Verification items for the finished model (mm, model axes). A direction names the side the tool comes from. Round coordinates to 2 decimals unless told otherwise and drop trailing zeros. Write each loop counter-clockwise with the first axis right and the second up, starting at its lowest first coordinate (ties: lowest second). Pieces come first, ordered by that corner, then holes. Notation, with made-up numbers: M 19.5,6.5 L 64.5,6.5 A21 ccw 64.5,36.5 Z; hole C 74,71 d11. An arc over 180 degrees is marked long. Write each question's results on one line, items separated by ' | '.
from build123d import *

# Parameters (mm, degrees)
SKETCH_1_R           = 4
EXTRUDE_1_DEPTH      = 11
SKETCH_2_R           = 3.01
CUT_EXTRUDE_2_DEPTH  = 2
SKETCH_3_R           = 2.5
CUT_EXTRUDE_3_DEPTH  = 4.3
SKETCH_4_W           = 2.01
SKETCH_4_H           = 4.01
CUT_EXTRUDE_4_DEPTH  = 0.7
SKETCH_5_R           = 2.5
CUT_EXTRUDE_5_DEPTH  = 1
SKETCH_7_R           = 4
CUT_EXTRUDE_6_DEPTH  = 10
SKETCH_12_R          = 3.25
CUT_EXTRUDE_7_DEPTH  = 2
SKETCH_13_R          = 4
SKETCH_13_R_2        = 2.5
EXTRUDE_2_DEPTH      = 2
CUT_EXTRUDE_START    = -3
SKETCH_14_R          = 4
SKETCH_14_R_2        = 2.5
CUT_EXTRUDE_8_DEPTH  = 3
SKETCH_15_R          = 7
SKETCH_15_R_2        = 5
EXTRUDE_3_DEPTH      = 14.9
EXTRUDE_START        = 7
SKETCH_16_R          = 7
SKETCH_16_R_2        = 4
EXTRUDE_4_DEPTH      = 7
SKETCH_17_R          = 0.8
CUT_EXTRUDE_10_DEPTH = 5
SKETCH_18_R          = 5
SKETCH_18_W          = 2.01
SKETCH_18_H          = 2.999191688
EXTRUDE_5_DEPTH      = 0.5
SKETCH_20_R          = 0.625
CUT_EXTRUDE_11_DEPTH = 9
CUT_EXTRUDE_START_2  = -9
SKETCH_21_R          = 7
CUT_EXTRUDE_12_DEPTH = 9
EXTRUDE_START_2      = -12.9
SKETCH_22_R          = 7.5
SKETCH_22_R_2        = 7
EXTRUDE_7_DEPTH      = 12.9
EXTRUDE_START_3      = -10
SKETCH_23_R          = 5
SKETCH_23_R_2        = 4.5
EXTRUDE_8_DEPTH      = 10


with BuildPart() as part:
    # Sketch 1 → Extrude 1 (new body)
    with BuildSketch(Plane(origin=(0, 0, 0), x_dir=(1, 0, 0), z_dir=(0, 1, 0))):
        with Locations(Location((0, 0, 0), (0, 0, 270))):
            Circle(SKETCH_1_R)
    extrude(amount=EXTRUDE_1_DEPTH)

    # Sketch 2 → Cut-Extrude 2 (cut)
    with BuildSketch(Plane.XZ):
        with Locations(Location((0, 0, 0), (0, 0, 270))):
            Circle(SKETCH_2_R)
    extrude(amount=-CUT_EXTRUDE_2_DEPTH, mode=Mode.SUBTRACT)

    # Sketch 3 → Cut-Extrude 3 (cut)
    with BuildSketch(Plane.XZ.offset(-2)):
        with Locations(Location((0, 0, 0), (0, 0, 270))):
            Circle(SKETCH_3_R)
    extrude(amount=-CUT_EXTRUDE_3_DEPTH, mode=Mode.SUBTRACT)

    # Sketch 4 → Cut-Extrude 4 (cut)
    with BuildSketch(Plane.XZ.offset(-6.3)):
        Rectangle(SKETCH_4_W, SKETCH_4_H)
    extrude(amount=-CUT_EXTRUDE_4_DEPTH, mode=Mode.SUBTRACT)

    # Sketch 5 → Cut-Extrude 5 (cut)
    with BuildSketch(Plane.XZ.offset(-7)):
        with Locations(Location((0, 0, 0), (0, 0, 270))):
            Circle(SKETCH_5_R)
    extrude(amount=-CUT_EXTRUDE_5_DEPTH, mode=Mode.SUBTRACT)

    # Sketch 7 → Cut-Extrude 6 (cut)
    with BuildSketch(Plane.XZ.offset(-8)):
        with Locations(Location((0, 0, 0), (0, 0, 270))):
            Circle(SKETCH_7_R)
    extrude(amount=-CUT_EXTRUDE_6_DEPTH, mode=Mode.SUBTRACT)

    # Sketch 12 → Cut-Extrude 7 (cut)
    with BuildSketch(Plane.XZ):
        with Locations(Location((0, 0, 0), (0, 0, 270))):
            Circle(SKETCH_12_R)
    extrude(amount=-CUT_EXTRUDE_7_DEPTH, mode=Mode.SUBTRACT)

    # Sketch 13 → Extrude 2 (add)
    with BuildSketch(Plane(origin=(0, 8, 0), x_dir=(1, 0, 0), z_dir=(0, 1, 0))):
        with Locations(Location((0, 0, 0), (0, 0, 270))):
            Circle(SKETCH_13_R)
        with Locations(Location((0, 0, 0), (0, 0, 90))):
            Circle(SKETCH_13_R_2, mode=Mode.SUBTRACT)
    extrude(amount=EXTRUDE_2_DEPTH)

    # Sketch 14 → Cut-Extrude 8 (cut)
    with BuildSketch(Plane(origin=(0, 10, 0), x_dir=(1, 0, 0), z_dir=(0, 1, 0)).offset(CUT_EXTRUDE_START)):
        with Locations(Location((0, 0, 0), (0, 0, 270))):
            Circle(SKETCH_14_R)
        with Locations(Location((0, 0, 0), (0, 0, 90))):
            Circle(SKETCH_14_R_2, mode=Mode.SUBTRACT)
    extrude(amount=CUT_EXTRUDE_8_DEPTH, mode=Mode.SUBTRACT)



with BuildPart() as body_2:
    # Sketch 15 → Extrude 3 (new body)
    with BuildSketch(Plane(origin=(0, 7, 0), x_dir=(1, 0, 0), z_dir=(0, 1, 0))):
        with Locations(Location((0, 0, 0), (0, 0, 270))):
            Circle(SKETCH_15_R)
        with Locations(Location((0, 0, 0), (0, 0, 270))):
            Circle(SKETCH_15_R_2, mode=Mode.SUBTRACT)
    extrude(amount=EXTRUDE_3_DEPTH)


with BuildPart() as part_1:
    add(part.part)

    add(body_2.part)  # Extrude 4 merges body 2
    # Sketch 16 → Extrude 4 (add)
    with BuildSketch(Plane.XZ.offset(-7).offset(EXTRUDE_START)):
        with Locations(Location((0, 0, 0), (0, 0, 90))):
            Circle(SKETCH_16_R)
        Circle(SKETCH_16_R_2, mode=Mode.SUBTRACT)
    extrude(amount=-EXTRUDE_4_DEPTH)

    # Sketch 17 → Cut-Extrude 10 (cut)
    with BuildSketch(Plane(origin=(0, 21.9, 0), x_dir=(1, 0, 0), z_dir=(0, 1, 0))):
        with Locations(Location((6, 0, 0), (0, 0, 270))):
            Circle(SKETCH_17_R)
        with Locations(Location((-6, 0, 0), (0, 0, 90))):
            Circle(SKETCH_17_R)
    extrude(amount=-CUT_EXTRUDE_10_DEPTH, mode=Mode.SUBTRACT)

    # Sketch 18 → Extrude 5 (add)
    with BuildSketch(Plane(origin=(0, 7, 0), x_dir=(1, 0, 0), z_dir=(0, 1, 0))):
        with Locations(Location((0, 0, 0), (0, 0, 180))):
            Circle(SKETCH_18_R)
        with Locations((0, 0.005404156)):
            Rectangle(SKETCH_18_W, SKETCH_18_H, mode=Mode.SUBTRACT)
    extrude(amount=EXTRUDE_5_DEPTH)

    # Sketch 20 → Cut-Extrude 11 (cut)
    with BuildSketch(Plane(origin=(0, 16.9, 0), x_dir=(1, 0, 0), z_dir=(0, 1, 0))):
        with Locations(Location((6, 0, 0), (0, 0, 270))):
            Circle(SKETCH_20_R)
        with Locations(Location((-6, 0, 0), (0, 0, 270))):
            Circle(SKETCH_20_R)
    extrude(amount=-CUT_EXTRUDE_11_DEPTH, mode=Mode.SUBTRACT)

    # Sketch 21 → Cut-Extrude 12 (cut)
    with BuildSketch(Plane(origin=(0, 21.9, 0), x_dir=(1, 0, 0), z_dir=(0, 1, 0)).offset(CUT_EXTRUDE_START_2)):
        with Locations(Location((0, 0, 0), (0, 0, 270))):
            Circle(SKETCH_21_R)
    extrude(amount=CUT_EXTRUDE_12_DEPTH, mode=Mode.SUBTRACT)

    # Sketch 22 → Extrude 7 (add)
    with BuildSketch(Plane(origin=(0, 12.9, 0), x_dir=(1, 0, 0), z_dir=(0, 1, 0)).offset(EXTRUDE_START_2)):
        with Locations(Location((0, 0, 0), (0, 0, 270))):
            Circle(SKETCH_22_R)
        Circle(SKETCH_22_R_2, mode=Mode.SUBTRACT)
    extrude(amount=EXTRUDE_7_DEPTH)

    # Sketch 23 → Extrude 8 (add)
    with BuildSketch(Plane(origin=(0, 12.9, 0), x_dir=(1, 0, 0), z_dir=(0, 1, 0)).offset(EXTRUDE_START_3)):
        Circle(SKETCH_23_R)
        with Locations(Location((0, 0, 0), (0, 0, 270))):
            Circle(SKETCH_23_R_2, mode=Mode.SUBTRACT)
    extrude(amount=EXTRUDE_8_DEPTH)


solid = part_1.part
1) Access from +Z, -Z, +X, -X, +Y, -Y to the whole of each face (thin tool, end or side, straight path). Record for faces 5 (the flat face through (-2, 0, 3)), 6 (the flat face through (-2, 2, -2)), 7 (the flat face through (-6, 7.9, 0)).
Calculated:
face 5: +Z, -Z, +X, -X, -Y | face 6: -Y | face 7: +Y
2) Depth check by flat-ended pin: P1, Ø2, axis at y = 3.5, z = 4, coming from the -X side; P2, Ø2, axis at y = 5.5, z = 5, coming from the -X side; P3, Ø1, axis at x = 4, y = 6, coming from the +Z side. Enter the tip coordinate at first touch or a pass-through.
Calculated:
P1: stops at x = -6.87 | P2: stops at x = -6.34 | P3: stops at z = 6.63
3) Sectioned sample at B-B, the plane y = 2.75. Record the cut outline in (x, z), and give its area (3 significant figures).
Calculated:
outline: C 0,0 d15; hole C 0,0 d5 | area: 157 mm²
4) Sectioned sample at D-D, the plane y = 12.25. Record the cut outline in (x, z) (3 decimals).
Calculated:
outline: C 0,0 d15; hole C -6,0 d1.25; hole C 0,0 d9; hole C 6,0 d1.25
5) Sectioned sample at C-C, the plane x = -6. Record the cut outline in (y, z) (3 decimals), and give its area (3 significant figures).
Calculated:
outline: M 0,-4.5 L 12.9,-4.5 L 12.9,-0.625 L 7.9,-0.625 L 7.9,0.625 L 12.9,0.625 L 12.9,4.5 L 0,4.5 Z | area: 110 mm²
6) Sectioned sample at A-A, the plane z = 0. Record the cut outline in (x, y) (3 decimals), and give its area (3 significant figures).
Calculated:
outline: M -7.5,0 L -3.25,0 L -3.25,2 L -2.5,2 L -2.5,6.3 L -1.005,6.3 L -1.005,7.5 L -4.5,7.5 L -4.5,12.9 L -5.375,12.9 L -5.375,7.9 L -6.625,7.9 L -6.625,12.9 L -7.5,12.9 Z; M 1.005,6.3 L 2.5,6.3 L 2.5,2 L 3.25,2 L 3.25,0 L 7.5,0 L 7.5,12.9 L 6.625,12.9 L 6.625,7.9 L 5.375,7.9 L 5.375,12.9 L 4.5,12.9 L 4.5,7.5 L 1.005,7.5 Z | area: 95.5 mm²
7) Draft check along X on faces 1 (the flat face through (1.005, 7, 0)), 2 (the flat face through (-3.4, 12.9, 3.2)), 3 (the cylindrical face through (0.33, 6.36, -7.493)), 4 (the cylindrical face through (-2.44, 4.12, 0.54)). Enter one of: pulls with the +X half, pulls with the -X half, needs draft (parallel to the pull), parting line crosses it, or undercut.
Calculated:
face 1: undercut | face 2: needs draft | face 3: parting line crosses it | face 4: undercut
8) Material ranges on line 1 (X direction, y = 9.4, z = 0) (3 decimals); line 2 (X direction, y = 10, z = 0.5) (3 decimals); line 3 (X direction, y = 5.25, z = 0), recorded low to high. Write a range as [from, to].
Calculated:
line 1: x = [-7.5, -6.625], [-5.375, -4.5], [4.5, 5.375], [6.625, 7.5] | line 2: x = [-7.483, -6.375], [-5.625, -4.472], [4.472, 5.625], [6.375, 7.483] | line 3: x = [-7.5, -2.5], [2.5, 7.5]
